```python
from build123d import *

# Parameters (mm, degrees)
SKETCH_1_W          = 10
SKETCH_1_H          = 10
SKETCH_1_W_2        = 8
SKETCH_1_H_2        = 8
EXTRUDE_1_DEPTH     = 495
SKETCH_3_R          = 2.1
CUT_EXTRUDE_2_DEPTH = 496.126246527
SKETCH_2_R          = 1.6
CUT_EXTRUDE_1_DEPTH = 496.126246527
SKETCH_7_R          = 1.6
CUT_EXTRUDE_4_DEPTH = 496.126246527
SKETCH_9_R          = 2.1
CUT_EXTRUDE_6_DEPTH = 496.126246527
CUT_EXTRUDE_7_REACH = 497.126
SKETCH_10_R         = 3
SKETCH_11_R         = 1.6
CUT_EXTRUDE_8_DEPTH = 496.126246527
SKETCH_12_R         = 1.6
CUT_EXTRUDE_9_DEPTH = 496.126246527


with BuildPart() as part:
    # ｽｹｯﾁ1 → 押し出し-薄板1 (new body)
    with BuildSketch(Plane.XY):
        Rectangle(SKETCH_1_W, SKETCH_1_H)
        Rectangle(SKETCH_1_W_2, SKETCH_1_H_2, mode=Mode.SUBTRACT)
    extrude(amount=EXTRUDE_1_DEPTH)

    # ｽｹｯﾁ3 → ｶｯﾄ - 押し出し2 (cut, through all)
    with BuildSketch(Plane(origin=(5, 0, 0), x_dir=(0, 0, -1), z_dir=(1, 0, 0))):
        with Locations(Location((-5, 0, 0), (0, 0, 90))):
            Circle(SKETCH_3_R)
    extrude(amount=-CUT_EXTRUDE_2_DEPTH, mode=Mode.SUBTRACT)

    # ｽｹｯﾁ2 → ｶｯﾄ - 押し出し1 (cut, through all)
    with BuildSketch(Plane(origin=(0, 5, 0), x_dir=(1, 0, 0), z_dir=(0, 1, 0))):
        with Locations(Location((0, -15, 0), (0, 0, 180))):
            Circle(SKETCH_2_R)
        with Locations(Location((0, -470, 0), (0, 0, 180))):
            Circle(SKETCH_2_R)
        with Locations(Location((0, -490, 0), (0, 0, 180))):
            Circle(SKETCH_2_R)
        with Locations(Location((0, -267.5, 0), (0, 0, 180))):
            Circle(SKETCH_2_R)
        with Locations(Location((0, -287.5, 0), (0, 0, 180))):
            Circle(SKETCH_2_R)
    extrude(amount=-CUT_EXTRUDE_1_DEPTH, mode=Mode.SUBTRACT)

    # ｽｹｯﾁ7 → ｶｯﾄ - 押し出し4 (cut, through all)
    with BuildSketch(Plane(origin=(5, 0, 0), x_dir=(0, 0, -1), z_dir=(1, 0, 0))):
        with Locations(Location((-475, 0, 0), (0, 0, 90))):
            Circle(SKETCH_7_R)
        with Locations(Location((-465, 0, 0), (0, 0, 90))):
            Circle(SKETCH_7_R)
    extrude(amount=-CUT_EXTRUDE_4_DEPTH, mode=Mode.SUBTRACT)

    # ｽｹｯﾁ9 → ｶｯﾄ - 押し出し6 (cut, through all)
    with BuildSketch(Plane(origin=(5, 0, 0), x_dir=(0, 0, -1), z_dir=(1, 0, 0))):
        with Locations(Location((-345, 0, 0), (0, 0, 90))):
            Circle(SKETCH_9_R)
        with Locations(Location((-150, 0, 0), (0, 0, 270))):
            Circle(SKETCH_9_R)
    extrude(amount=-CUT_EXTRUDE_6_DEPTH, mode=Mode.SUBTRACT)

    # ｽｹｯﾁ10 → ｶｯﾄ - 押し出し7 (cut, up to next)
    with BuildSketch(Plane(origin=(0, 5, 0), x_dir=(1, 0, 0), z_dir=(0, 1, 0)), mode=Mode.PRIVATE) as cut_extrude_7_sk1:
        with Locations(Location((0, -287.5, 0), (0, 0, 180))):
            Circle(SKETCH_10_R)
    cut_extrude_7_tool1 = extrude(cut_extrude_7_sk1.sketch, amount=-CUT_EXTRUDE_7_REACH, mode=Mode.PRIVATE) & part.part
    add(cut_extrude_7_tool1.solids().sort_by_distance((0, 5, 287.5))[0], mode=Mode.SUBTRACT)

    # ｽｹｯﾁ11 → ｶｯﾄ - 押し出し8 (cut, through all)
    with BuildSketch(Plane.XZ.offset(5)):
        with Locations((0, 180)):
            Circle(SKETCH_11_R)
        with Locations((0, 200)):
            Circle(SKETCH_11_R)
        with Locations((0, 220)):
            Circle(SKETCH_11_R)
    extrude(amount=-CUT_EXTRUDE_8_DEPTH, mode=Mode.SUBTRACT)

    # ｽｹｯﾁ12 → ｶｯﾄ - 押し出し9 (cut, through all)
    with BuildSketch(Plane.XZ.offset(5)):
        with Locations((0, 127.5)):
            Circle(SKETCH_12_R)
        with Locations((0, 107.5)):
            Circle(SKETCH_12_R)
    extrude(amount=-CUT_EXTRUDE_9_DEPTH, mode=Mode.SUBTRACT)


solid = part.part
```
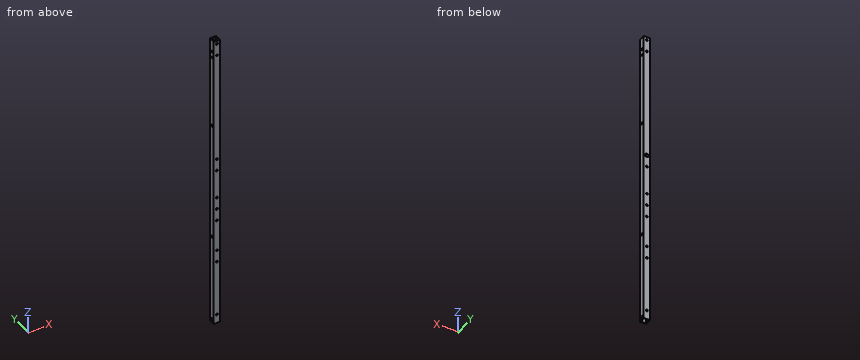
Verification items for the finished model (mm, model axes). Round coordinates to 2 decimals unless told otherwise and drop trailing zeros. Order: outer loops, then holes, each group sorted by start corner. A loop starts at its lowest first (then second) coordinate and runs counter-clockwise, first axis right, second up. Notation, with made-up numbers: (44, 10.25) - (90, 10.25) arc R22 ccw to (90, 43.25) - close; hole circle Ø1 at (6.25, 76). An arc over 180 degrees is marked (long way). Use CSV: the item, a comma, the result in double quotes. Start each with the question number.
1) Thickness scan on L1, parallel to Z at x = -4.75, y = 0; L2, parallel to X at y = 0.5, z = 455.5; L3, parallel to Z at x = 4.75, y = -0.5. Record the ranges inside material, lowest first.
2) Section check A-A, the plane z = 402. Record the cut outline in (x, y), plus the area to 3 significant figures.
3) Section check B-B, the plane x = 0. State how many separate pieces and enclosed holes the cut face has, plus the area to 3 significant figures.
Answers:
1,L1,"z = 0 to 2.9, 7.1 to 147.9, 152.1 to 342.9, 347.1 to 463.4, 466.6 to 473.4, 476.6 to 495"
1,L2,"x = -5 to -4, 4 to 5"
1,L3,"z = 0 to 2.96, 7.04 to 147.96, 152.04 to 342.96, 347.04 to 463.48, 466.52 to 473.48, 476.52 to 495"
2,outline,"(-5, -5) - (5, -5) - (5, 5) - (-5, 5) - close; hole (-4, -4) - (4, -4) - (4, 4) - (-4, 4) - close"
2,area,"36.0 mm²"
3,separate pieces,"22"
3,enclosed holes,"0"
3,area,"923 mm²"
